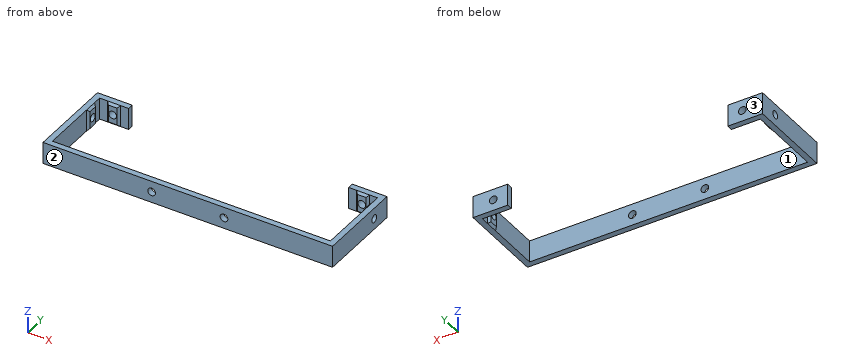
```python
from build123d import *

# Parameters (mm, degrees)
F1_DEPTH  = 15
F3_DEPTH  = 15
F4_SIZE   = 1.5
F5_R      = 2.65
F6_DEPTH  = 4
F7_R      = 2.65
F8_DEPTH  = 200.001
F9_R      = 2.65
F10_DEPTH = 5.5


with BuildPart() as f1:
    # F0 (on Top) → F1 (new body)
    with BuildSketch(Plane.XY):
        Polygon((0, 60), (0, 0), (200, 0), (200, 60), (176, 60), (176, 56), (196, 56), (196, 4), (4, 4), (4, 56), (24, 56), (24, 60), align=None)
    extrude(amount=F1_DEPTH)

    # F2 (on Top) → F3 (join, through all)
    with BuildSketch(Plane.XY):
        Polygon((17, 54.5), (18.5, 56), (9.5, 56), (11, 54.5), align=None)
        Polygon((5.5, 49), (4, 50.5), (4, 41.5), (5.5, 43), align=None)
        Polygon((196, 41.5), (196, 50.5), (194.5, 49), (194.5, 43), align=None)
        Polygon((189, 54.5), (190.5, 56), (181.5, 56), (183, 54.5), align=None)
    extrude(amount=F3_DEPTH)

    # F4
    f4_edges = [f1.edges().sort_by_distance(p)[0] for p in [
        (5.5, 46, 15),
        (5.5, 46, 0),
        (14, 54.5, 0),
        (14, 54.5, 15),
        (186, 54.5, 15),
        (194.5, 46, 15),
        (194.5, 46, 0),
        (186, 54.5, 0),
    ]]
    chamfer(f4_edges, length=F4_SIZE)

    # F5 (on face) → F6 (cut, through all)
    with BuildSketch(Plane.XZ):
        with Locations((75, 7.5)):
            Circle(F5_R)
        with Locations((125, 7.5)):
            Circle(F5_R)
    extrude(amount=-F6_DEPTH, mode=Mode.SUBTRACT)

    # F7 (on face) → F8 (cut, through all)
    with BuildSketch(Plane.YZ.offset(200)):
        with Locations((46, 7.5)):
            Circle(F7_R)
    extrude(amount=-F8_DEPTH, mode=Mode.SUBTRACT)

    # F9 (on face) → F10 (cut, through all)
    with BuildSketch(Plane(origin=(0, 60, 0), x_dir=(-1, 0, 0), z_dir=(0, 1, 0))):
        with Locations((-186, 7.5)):
            Circle(F9_R)
        with Locations((-14, 7.5)):
            Circle(F9_R)
    extrude(amount=-F10_DEPTH, mode=Mode.SUBTRACT)


solid = f1.part
```
Verification items for the finished model (mm, model axes). Face numbers are marked on the shaded views. Coordinates: 2 decimals unless noted, no trailing zeros. Loops run counter-clockwise (first coordinate to the right, second up) from the corner with the lowest first, then second, coordinate; pieces in that order, holes last. Notation, with made-up numbers: (55.5, 22.5) -> (83.5, 22.5) arc R9 ccw to (83.5, 27.5) -> close; hole circle Ø9 at (77, 69.5). An arc over 180 degrees is marked (long way). Put each result on its own line as item: value.
1. Mould release check, pull along Y, two halves, no side actions. Record for the marked faces 1, 2 and 3: pulls with the +Y half, pulls with the -Y half, needs draft (parallel to the pull), parting line crosses it, or undercut.
Result set:
face 1: undercut
face 2: pulls with the -Y half
face 3: pulls with the +Y half
2. Section check B-B, the plane x = 125. Record the boundary of the cut face in (y, z).
Result set:
outline: (0, 0) -> (4, 0) -> (4, 4.85) -> (0, 4.85) -> close; (0, 10.15) -> (4, 10.15) -> (4, 15) -> (0, 15) -> close
3. Gauge pin test, flat ends, axial feed: P1, Ø8, axis at y = 16, z = 12, coming from the -X side; P2, Ø3, axis at x = 156, z = 5.5, coming from the +Y side; P3, Ø3, axis at y = 45.5, z = 8, coming from the -X side. Record the tip position at first contact, or that the pin passes through.
Result set:
P1: stops at x = 0
P2: stops at y = 4
P3: passes through
4. Thickness scan on line 1 (X direction, y = 41.5, z = 12.25); line 2 (X direction, y = 57, z = 12); line 3 (Z direction, x = 75, y = 2.05). Record the ranges inside material, lowest first.
Result set:
line 1: x = 0 to 4, 196 to 200
line 2: x = 0 to 24, 176 to 200
line 3: z = 0 to 4.85, 10.15 to 15
5. Section check D-D, the plane x = 14. Record the boundary of the cut face in (y, z), then the cut area to 3 significant figures.
Result set:
outline: (0, 0) -> (4, 0) -> (4, 15) -> (0, 15) -> close; (54.5, 1.5) -> (56, 0) -> (60, 0) -> (60, 4.85) -> (54.5, 4.85) -> close; (54.5, 10.15) -> (60, 10.15) -> (60, 15) -> (56, 15) -> (54.5, 13.5) -> close
area: 111 mm^2
6. Section check A-A, the plane y = 13. Record the boundary of the cut face in (x, z).
Result set:
outline: (0, 0) -> (4, 0) -> (4, 15) -> (0, 15) -> close; (196, 0) -> (200, 0) -> (200, 15) -> (196, 15) -> close
7. Section check C-C, the plane y = 46. Record the boundary of the cut face in (x, z).
Result set:
outline: (0, 0) -> (4, 0) -> (5.5, 1.5) -> (5.5, 4.85) -> (0, 4.85) -> close; (0, 10.15) -> (5.5, 10.15) -> (5.5, 13.5) -> (4, 15) -> (0, 15) -> close; (194.5, 1.5) -> (196, 0) -> (200, 0) -> (200, 4.85) -> (194.5, 4.85) -> close; (194.5, 10.15) -> (200, 10.15) -> (200, 15) -> (196, 15) -> (194.5, 13.5) -> close
